Verification items for the finished model (mm, model axes). A direction names the side the tool comes from. Coordinates: 2 decimals unless noted, no trailing zeros. Loops run counter-clockwise (first coordinate to the right, second up) from the corner with the lowest first, then second, coordinate; pieces in that order, holes last.
Q1. Mould release check, pull along X, two halves, no side actions. Record for faces 4 (the face through (-9.07, 26, 1)), 5 (the face through (47.93, 0, 0)), 6 (the face through (35, -2, 1)), 7 (the face through (-5, -5, 1)): +X half, -X half, draft (parallel to the pull), parting line (faces both ways), or undercut.
Q2. Go/stop test with flat-tipped pins: P1, Ø1.5, axis at x = 6.5, z = 0.5, coming from the -Y side; P2, Ø4, axis at x = 2, z = -1.5, coming from the +Y side; P3, Ø16, axis at x = 9, y = 41, coming from the +Z side; P4, Ø2.5, axis at x = 47, z = 2.5, coming from the +Y side. Record where each tip stops, or that it passes through.
Q3. Sectioned sample at A-A (y = 32). Enter the section's corners in (x, z).
Q4. Material ranges on probe 1 along X at (y, z) = (2.5, 1); probe 2 along X at (y, z) = (0, -2.5); probe 3 along X at (y, z) = (15.5, -1.5), recorded low to high.
Q5. Sectioned sample at B-B (z = -3). Enter the section's corners in (x, y).
Q6. Sectioned sample at D-D (y = 2). Enter the section's corners in (x, z).
Q7. Access from +Z, -Z, +X, -X, +Y, -Y to the whole of each face (thin tool, end or side, straight path). Record for faces 1 (the face through (46, 5, 1)), 2 (the face through (13.2, 22.5, 5)), 3 (the face through (0, 15, 0)).
Q8. Sectioned sample at C-C (x = -2). Enter the section's corners in (y, z), then the cut area to 3 significant figures.
Autodesk Inventor part; units mm, degrees
ref_plane "Plano de trabajo1" through (0, 0, 16) normal (0, 0, 1) x (1, 0, 0)
ref_plane "YZ Plane" through (0, 0, 0) normal (1, 0, 0) x (0, 1, 0)
ref_plane "XZ Plane" through (0, 0, 0) normal (0, 1, 0) x (-1, 0, 0)
sketch "Boceto1" plane through (0, 0, 0) normal (0, 0, 1) x (1, 0, 0)
  line L0 (-9.0701, 0) -> (44.9299, 0)
  line L1 (44.9299, 0) -> (-9.0701, 54)
  line L2 (-9.0701, 0) -> (-9.0701, 54)
  point P0 (0, 0)
  dimension "d0" = 54
  dimension "d2" = 45
extrude "Extrusión1" add sketch "Boceto1" along normal blind 5
sketch "Boceto2" plane through (0, 0, 5) normal (0, 0, 1) x (1, 0, 0)
  line L0 (44.9299, 0) -> (-9.0701, 54)
  line L1 (44.9299, 5) -> (47.9299, 5)
  line L2 (47.9299, 5) -> (47.9299, 0)
  line L3 (47.9299, 0) -> (44.9299, 0)
  line L4 (44.9299, 0) -> (44.9299, 5)
  point P0 (0, 0)
  dimension "d9" = 3
  dimension "d10" = 5
extrude "Extrusión2" add sketch "Boceto2" against normal blind 9
sketch "Boceto4" plane through (0, 0, 0) normal (0, 0, -1) x (-1, 0, 0)
  line L0 (-48.0778, 0) -> (35.3608, 0) construction
  line L1 (-47.9299, 5) -> (-47.9299, 0)
  line L2 (-47.9299, 0) -> (9.0701, 57)
  line L3 (-47.9299, 0) -> (40.6563, 0) construction
  line L4 (9.0701, 0) -> (9.0701, 57)
  line L5 (9.0701, 0) -> (-47.9299, 0)
  point P0 (0, 0)
  dimension "d24" = 45
extrude "Extrusión3" add sketch "Boceto4" along normal blind 4
sketch "Boceto5" plane through (0, 0, -4) normal (0, 0, -1) x (-1, 0, 0)
  line L0 (0, 0) -> (0, 35)
  line L1 (0, 35) -> (-35, 0)
  line L2 (0, 35) -> (67.1316, 35) construction
  line L3 (0, 0) -> (-35, 0)
  line L4 (9.0701, 0) -> (-44.9299, 0)
  dimension "d19" = 35
  dimension "d20" = 135
extrude "Extrusión4" cut sketch "Boceto5" against normal blind 15
sketch "Boceto6" plane through (-9.0701, 0, -4) normal (0, -1, 0) x (1, 0, 0)
  line L0 (9.0701, 0) -> (9.0701, 9)
  line L1 (9.0701, 9) -> (0, 9)
  line L2 (0, 9) -> (0, 0)
  line L3 (0, 0) -> (9.0701, 0)
  line L4 (9.0701, 0) -> (9.0701, 9)
  point P0 (9.0701, 4)
extrude "Extrusión5" add sketch "Boceto6" along normal blind 5
sketch "Boceto7" plane through (44.9299, 0, 5) normal (0, -1, 0) x (1, 0, 0)
  line L0 (-9.9299, -9) -> (-44.9299, -9)
  line L1 (3, 0) -> (0, 0)
  line L2 (-9.9299, -9) -> (3, -9)
  line L3 (3, -9) -> (3, 0)
  line L4 (3, 0) -> (-9.9299, 0)
  line L5 (-9.9299, 0) -> (-9.9299, -9)
  point P0 (-44.9299, -5)
extrude "Extrusión6" add sketch "Boceto7" along normal blind 5
ref_plane "Plano de trabajo1" through (0, 0, 16) normal (0, 0, 1) x (1, 0, 0)
properties part number "BaseBeamSplitter-D" material "Plástico ABS"
Geometry check:
1. face 4: -X half
1. face 5: +X half
1. face 6: undercut
1. face 7: draft
2. P1: stops at y = 27.75
2. P2: stops at y = 47.93
2. P3: stops at z = 5
2. P4: stops at y = 5
3. outline: (-9.07, -4) - (0, -4) - (0, 5) - (-9.07, 5) - close; (3, -4) - (15.93, -4) - (15.93, 0) - (12.93, 0) - (12.93, 5) - (3, 5) - close
4. probe 1: x = -9.07 to 0, 32.5 to 42.43, 44.93 to 47.93
4. probe 2: x = -9.07 to 0, 35 to 47.93
4. probe 3: x = -9.07 to 0, 19.5 to 32.43
5. outline: (-9.07, -5) - (0, -5) - (0, 35) - (35, 0) - (35, -5) - (47.93, -5) - (47.93, 5) - (44.93, 5) - (44.93, 3) - (-9.07, 57) - close
6. outline: (-9.07, -4) - (0, -4) - (0, 5) - (-9.07, 5) - close; (33, -4) - (47.93, -4) - (47.93, 5) - (44.93, 5) - (44.93, 0) - (42.93, 0) - (42.93, 5) - (33, 5) - close
7. face 1: +Z, -Z, +X, +Y
7. face 2: +Z, +X, -X, +Y, -Y
7. face 3: +Z, -Z, -Y
8. outline: (-5, -4) - (49.93, -4) - (49.93, 0) - (46.93, 0) - (46.93, 5) - (-5, 5) - close
8. area: 479 mm2
